Source: CAD feature listing. Evaluate the final solid. Frame: model axes, mm. Face numbers are marked on the shaded views. A direction names the side the tool comes from. Give positions to 0.01 mm unless a question says otherwise; leave off trailing zeros. Write each loop counter-clockwise with the first axis right and the second up, starting at its lowest first coordinate (ties: lowest second). Pieces come first, ordered by that corner, then holes. Notation, with made-up numbers: (72, 56.25) -> (95, 56.25) arc R30 cw to (95, 95.25) -> close; hole circle Ø2 at (80.5, 58.25). An arc over 180 degrees is marked (long way). Write item = value, one per line.
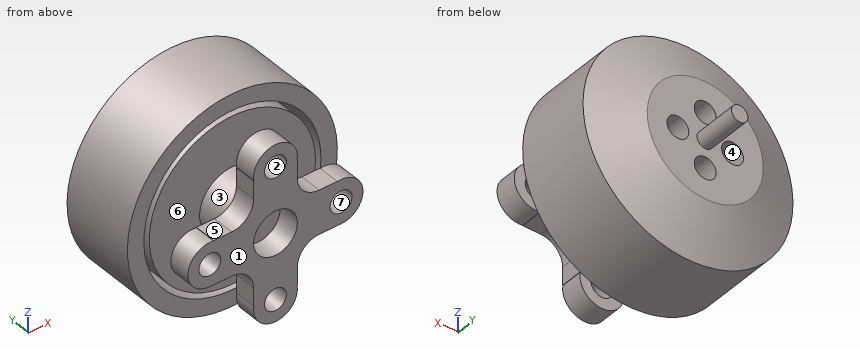
from build123d import *

# Parameters (mm, degrees)
SKETCH1_R           = 2
SKETCH1_R_2         = 1
BOSS_EXTRUDE1_DEPTH = 2
FILLET1_R           = 2
SKETCH2_R           = 3
BOSS_EXTRUDE2_DEPTH = 3
SKETCH3_R           = 9.6
BOSS_EXTRUDE3_DEPTH = 9
SKETCH4_R           = 0.75
BOSS_EXTRUDE4_DEPTH = 4
SKETCH5_R           = 1
CUT_EXTRUDE1_DEPTH  = 4
CHAMFER1_SIZE       = 2
CHAMFER1_SIZE2      = 4.289013841
CUT_EXTRUDE2_REACH  = 20.797
SKETCH6_R           = 8.1
SKETCH6_R_2         = 7.6


with BuildPart() as part:
    # Sketch1 → Boss-Extrude1 (new body)
    with BuildSketch(Plane(origin=(0, 0, 0), x_dir=(1, 0, 0), z_dir=(0, 1, 0))):
        with BuildLine():
            Line((-5.656854249, -2), (-2, -2))
            Line((-2, -2), (-2, -5.656854249))
            ThreePointArc((-2, -5.656854249), (-1.986019357, -5.661777734), (-1.972026594, -5.666666667))
            ThreePointArc((-1.972026594, -5.666666667), (0, -8), (1.972026594, -5.666666667))
            ThreePointArc((1.972026594, -5.666666667), (1.986019357, -5.661777734), (2, -5.656854249))
            Line((2, -5.656854249), (2, -2))
            Line((2, -2), (5.656854249, -2))
            ThreePointArc((5.656854249, -2), (5.661777734, -1.986019357), (5.666666667, -1.972026594))
            ThreePointArc((5.666666667, -1.972026594), (8, 0), (5.666666667, 1.972026594))
            ThreePointArc((5.666666667, 1.972026594), (5.661777734, 1.986019357), (5.656854249, 2))
            Line((5.656854249, 2), (2, 2))
            Line((2, 2), (2, 5.656854249))
            ThreePointArc((2, 5.656854249), (1.986019357, 5.661777734), (1.972026594, 5.666666667))
            ThreePointArc((1.972026594, 5.666666667), (0, 8), (-1.972026594, 5.666666667))
            ThreePointArc((-1.972026594, 5.666666667), (-1.986019357, 5.661777734), (-2, 5.656854249))
            Line((-2, 5.656854249), (-2, 2))
            Line((-2, 2), (-5.656854249, 2))
            ThreePointArc((-5.656854249, 2), (-5.661777734, 1.986019357), (-5.666666667, 1.972026594))
            ThreePointArc((-5.666666667, 1.972026594), (-8, 0), (-5.666666667, -1.972026594))
            ThreePointArc((-5.666666667, -1.972026594), (-5.661777734, -1.986019357), (-5.656854249, -2))
        make_face()
        with Locations(Location((0, 0, 0), (0, 0, 270))):
            Circle(SKETCH1_R, mode=Mode.SUBTRACT)
        with Locations(Location((6, 0, 0), (0, 0, 270))):
            Circle(SKETCH1_R_2, mode=Mode.SUBTRACT)
        with Locations(Location((0, 6, 0), (0, 0, 270))):
            Circle(SKETCH1_R_2, mode=Mode.SUBTRACT)
        with Locations(Location((-6, 0, 0), (0, 0, 270))):
            Circle(SKETCH1_R_2, mode=Mode.SUBTRACT)
        with Locations(Location((0, -6, 0), (0, 0, 270))):
            Circle(SKETCH1_R_2, mode=Mode.SUBTRACT)
    extrude(amount=BOSS_EXTRUDE1_DEPTH)

    # Fillet1
    fillet1_edges = [part.edges().sort_by_distance(p)[0] for p in [
        (2, 1, 2),
        (-2, 1, 2),
        (-2, 1, -2),
        (2, 1, -2),
    ]]
    fillet(fillet1_edges, radius=FILLET1_R)

    # Sketch2 → Boss-Extrude2 (add)
    with BuildSketch(Plane(origin=(0, 2, 0), x_dir=(1, 0, 0), z_dir=(0, 1, 0))):
        with Locations(Location((0, 0, 0), (0, 0, 270))):
            Circle(SKETCH2_R)
    extrude(amount=BOSS_EXTRUDE2_DEPTH)

    # Sketch3 → Boss-Extrude3 (add)
    with BuildSketch(Plane(origin=(0, 5, 0), x_dir=(1, 0, 0), z_dir=(0, 1, 0))):
        with Locations(Location((0, 0, 0), (0, 0, 270))):
            Circle(SKETCH3_R)
    extrude(amount=BOSS_EXTRUDE3_DEPTH)

    # Sketch4 → Boss-Extrude4 (add)
    with BuildSketch(Plane(origin=(0, 14, 0), x_dir=(1, 0, 0), z_dir=(0, 1, 0))):
        with Locations(Location((0, 0, 0), (0, 0, 270))):
            Circle(SKETCH4_R)
    extrude(amount=BOSS_EXTRUDE4_DEPTH)

    # Sketch5 → Cut-Extrude1 (cut)
    with BuildSketch(Plane(origin=(0, 14, 0), x_dir=(1, 0, 0), z_dir=(0, 1, 0))):
        with Locations(Location((-2.5, 0, 0), (0, 0, 270))):
            Circle(SKETCH5_R)
        with Locations(Location((0, 2.5, 0), (0, 0, 270))):
            Circle(SKETCH5_R)
        with Locations(Location((2.5, 0, 0), (0, 0, 270))):
            Circle(SKETCH5_R)
        with Locations(Location((0, -2.5, 0), (0, 0, 270))):
            Circle(SKETCH5_R)
    extrude(amount=-CUT_EXTRUDE1_DEPTH, mode=Mode.SUBTRACT)

    # Chamfer1
    chamfer1_edges = [part.edges().sort_by_distance(p)[0] for p in [
        (0, 14, -9.6),
    ]]
    chamfer1_side = [part.faces().sort_by_distance(p)[0] for p in [
        (0, 9.5, -9.6),
    ]]
    chamfer(chamfer1_edges, length=CHAMFER1_SIZE, length2=CHAMFER1_SIZE2, reference=chamfer1_side[0])

    # Cut-Extrude2: up to this cone (the profile starts inside it)
    cut_extrude2_end = Plane(origin=(0, 5, 0), z_dir=(0, -1, 0)).offset(-9.82148564) * Cone(2.145e-06, 111.901942411, 52.180731709, align=(Align.CENTER, Align.CENTER, Align.MIN), mode=Mode.PRIVATE)
    # Sketch6 → Cut-Extrude2 (cut, up to the surface)
    with BuildSketch(Plane.XZ.offset(-5), mode=Mode.PRIVATE) as cut_extrude2_sk1:
        with Locations(Location((0, 0, 0), (0, 0, 270))):
            Circle(SKETCH6_R)
        with Locations(Location((0, 0, 0), (0, 0, 270))):
            Circle(SKETCH6_R_2, mode=Mode.SUBTRACT)
    cut_extrude2_tool1 = extrude(cut_extrude2_sk1.sketch, amount=-CUT_EXTRUDE2_REACH, mode=Mode.PRIVATE) & cut_extrude2_end
    add(cut_extrude2_tool1.solids().sort_by_distance((0, 5, 7.870897))[0], mode=Mode.SUBTRACT)


solid = part.part
1) Material intervals for L1, parallel to X at y = 6.5, z = 0; L2, parallel to Z at x = -2.5, y = 7; L3, parallel to Z at x = -3.75, y = 7.25, sorted ascending.
Computed:
L1 = -9.6 to -8.1, -7.6 to 7.6, 8.1 to 9.6
L2 = -9.27 to -7.7, -7.18 to 7.18, 7.7 to 9.27
L3 = -8.84 to -7.18, -6.61 to 6.61, 7.18 to 8.84
2) Draft query along X for the marked faces 1, 2 and 3. Return one class per face: pulls with the +X half, pulls with the -X half, needs draft (parallel to the pull), parting line crosses it, or undercut.
Computed:
face_1 = needs draft
face_2 = undercut
face_3 = parting line crosses it
3) Cut plane C-C (y = 15). Return the cut outline in (x, z), then the cut area to 3 significant figures.
Computed:
outline = circle Ø1.5 at (0, 0)
area = 1.77 mm²
4) Cut plane A-A (x = 0). State how many separate pieces and enclosed holes the cut face has, then the cut area to 3 significant figures.
Computed:
separate_pieces = 3
enclosed_holes = 0
area = 182 mm²
5) Contact query for flat-ended pins moving along their axis: pin 1 (10 mm diameter, centred on y = 15, z = -3, fed in from -X); pin 2 (0.5 mm diameter, centred on y = 1, z = -5, fed in from -X); pin 3 (3 mm diameter, centred on x = -2.5, z = 0, fed in from +Y); pin 4 (1.3 mm diameter, centred on x = -5, y = 0.5, fed in from +Z). Output: stop coordinate, or through.
Computed:
pin_1 = -9.6
pin_2 = -2
pin_3 = 14
pin_4 = 2
6) Access query for the marked faces 4, 5, 6 and 7. Directions: +Z, -Z, +X, -X, +Y, -Y. A direction counts if a zero-diameter tool reaches every point of the face in a straight line with its end or side. Return the directions, or none.
Computed:
face_4 = +Y
face_5 = +Z, -X, -Y
face_6 = none
face_7 = -Y
